from build123d import *

# Parameters (mm, degrees)
BOSS_EXTRUDE1_DEPTH      = 20
BOSS_EXTRUDE2_REACH      = 36.375
BOSS_EXTRUDE2_END_RADIUS = 102
BOSS_EXTRUDE2_START      = -9
SKETCH3_W                = 10
SKETCH3_H                = 2.5
SKETCH4_W                = 10
SKETCH4_H                = 2
BOSS_EXTRUDE3_DEPTH      = 10
CHAMFER2_SIZE            = 3
CHAMFER2_SIZE2           = 1.732050808
CHAMFER1_SIZE            = 4
CHAMFER1_SIZE2           = 2.309401077
SKETCH6_W                = 10
SKETCH6_H                = 1
BOSS_EXTRUDE4_DEPTH      = 0.2
CHAMFER3_SIZE            = 0.5


with BuildPart() as part:
    # Sketch2 → Boss-Extrude1 (new body)
    with BuildSketch(Plane(origin=(0, 0, 0), x_dir=(1, 0, 0), z_dir=(0, 1, 0))):
        with BuildLine():
            Line((-15.3, 1.977371993), (-15, 0))
            ThreePointArc((-15, 0), (0, 1.131400334), (15, 0))
            Line((15, 0), (15.3, 1.977371993))
            ThreePointArc((15.3, 1.977371993), (0, 3.131400334), (-15.3, 1.977371993))
        make_face()
    extrude(amount=BOSS_EXTRUDE1_DEPTH)

    # Boss-Extrude2: up to this cylinder (the profile starts outside it)
    boss_extrude2_end = Plane(origin=(0, 6.463137, 98.868599666), z_dir=(0, -1, 0)) * Cylinder(BOSS_EXTRUDE2_END_RADIUS, 277.75, mode=Mode.PRIVATE)
    # Sketch3 → Boss-Extrude2 (add, up to the surface)
    with BuildSketch(Plane.XY.offset(BOSS_EXTRUDE2_START), mode=Mode.PRIVATE) as boss_extrude2_sk1:
        with Locations((0, 6.463137396)):
            Rectangle(SKETCH3_W, SKETCH3_H)
    boss_extrude2_tool1 = extrude(boss_extrude2_sk1.sketch, amount=BOSS_EXTRUDE2_REACH, mode=Mode.PRIVATE) - boss_extrude2_end
    add(boss_extrude2_tool1.solids().sort_by_distance((0, 6.463137, -9))[0])

    # Sketch4 → Boss-Extrude3 (add)
    with BuildSketch(Plane(origin=(0, 7.713137396, 0), x_dir=(1, 0, 0), z_dir=(0, 1, 0))):
        with Locations((0, 8)):
            Rectangle(SKETCH4_W, SKETCH4_H)
    extrude(amount=BOSS_EXTRUDE3_DEPTH)

    # Chamfer2
    chamfer2_edges = [part.edges().sort_by_distance(p)[0] for p in [
        (0, 7.713137396, -7),
    ]]
    chamfer2_side = [part.faces().sort_by_distance(p)[0] for p in [
        (0, 12.713137396, -7),
    ]]
    chamfer(chamfer2_edges, length=CHAMFER2_SIZE, length2=CHAMFER2_SIZE2, reference=chamfer2_side[0])

    # Chamfer1
    chamfer1_edges = [part.edges().sort_by_distance(p)[0] for p in [
        (0, 5.213137396, -9),
    ]]
    chamfer1_side = [part.faces().sort_by_distance(p)[0] for p in [
        (0, 11.463137396, -9),
    ]]
    chamfer(chamfer1_edges, length=CHAMFER1_SIZE, length2=CHAMFER1_SIZE2, reference=chamfer1_side[0])

    # Sketch6 → Boss-Extrude4 (add)
    with BuildSketch(Plane.XY.offset(-7)):
        with Locations((0, 13.213137396)):
            Rectangle(SKETCH6_W, SKETCH6_H)
    extrude(amount=BOSS_EXTRUDE4_DEPTH)

    # Chamfer3
    # the kernel refuses this chamfer: 0.5 mm, written as the material it takes off along each edge
    with BuildSketch(Plane(origin=(-6.285841494, 13.713137396, -6.8), x_dir=(0, 0.027495876610585647, -0.9996219169112968), z_dir=(1, 0, 0))) as chamfer3_piece_1_section:
        Polygon((CHAMFER3_SIZE * 0.999621916911, -CHAMFER3_SIZE * 0.0274958766106), (-CHAMFER3_SIZE * 0.0274958766106, -CHAMFER3_SIZE * 0.999621916911), (0, 0), align=None)
    chamfer3_piece_1 = extrude(amount=12.571682988, mode=Mode.PRIVATE)
    chamfer3_piece_1 = split(chamfer3_piece_1, bisect_by=Plane(origin=(0, 13.506192151, -7), z_dir=(0, 0, 1)), keep=Keep.TOP, mode=Mode.PRIVATE)
    add(chamfer3_piece_1, mode=Mode.SUBTRACT)


solid = part.part
Source: CAD feature listing. Evaluate the final solid. Frame: model axes, mm. A direction names the side the tool comes from. Coordinates: 2 decimals unless noted, no trailing zeros. Order: outer loops, then holes, each group sorted by start corner. A loop starts at its lowest first (then second) coordinate and runs counter-clockwise, first axis right, second up.
Item 1: Cut plane A-A (y = 15). Return loops of the section in (x, z).
Output values:
outline: (-15.3, -1.98) arc R102 ccw to (15.3, -1.98) - (15, 0) arc R100 cw to (-15, 0) - close; (-5, -9) - (5, -9) - (5, -7) - (-5, -7) - close
Item 2: Material intervals for line 1 (Z direction, x = -1, y = 13.5); line 2 (Y direction, x = 1, z = -5.25); line 3 (X direction, y = 7.5, z = -4.75), sorted ascending.
Output values:
line 1: z = -9 to -7, -3.13 to -1.13
line 2: y = 5.21 to 7.71
line 3: x = -5 to 5
Item 3: Set-up query: faces 1 (the face through (-15.15, 9.86, -1)), 2 (the face through (5, 10, -7)), 3 (the face through (0, 17.713, -8)), 4 (the face through (0, 16, -7)). Return all of +Z, -Z, +X, -X, +Y, -Y with unobstructed straight access to the full face (end or side cutting, diameter ignored); none if empty.
Output values:
face 1: +Z, -X, +Y, -Y
face 2: -Z, +X, +Y, -Y
face 3: -Z, +X, -X, +Y
face 4: +X, -X, +Y
Item 4: Pull-direction query (Y, two-part tool) for faces 5 (the face through (0, 12, -7)), 6 (the face through (-5, 10, -7)), 7 (the face through (0, 20, -2)); classes: pulls with the +Y half, pulls with the -Y half, needs draft (parallel to the pull), parting line crosses it, or undercut.
Output values:
face 5: undercut
face 6: needs draft
face 7: pulls with the +Y half
Item 5: Cut plane D-D (y = 4). Return loops of the section in (x, z).
Output values:
outline: (-15.3, -1.98) arc R102 ccw to (15.3, -1.98) - (15, 0) arc R100 cw to (-15, 0) - close
Item 6: Cut plane B-B (z = -0.75). Return loops of the section in (x, y), plus the area to 3 significant figures.
Output values:
outline: (-15.11, 0) - (-8.73, 0) - (-8.73, 20) - (-15.11, 20) - close; (8.73, 0) - (15.11, 0) - (15.11, 20) - (8.73, 20) - close
area: 256 mm2
Item 7: Cut plane C-C (x = -3.5). Return loops of the section in (y, z), plus the area to 3 significant figures.
Output values:
outline: (0, -3.07) - (5.21, -3.07) - (5.21, -6.69) - (9.21, -9) - (17.71, -9) - (17.71, -7) - (13.41, -7) - (13.21, -6.8) - (12.71, -6.8) - (12.71, -7) - (10.71, -7) - (7.71, -5.27) - (7.71, -3.07) - (20, -3.07) - (20, -1.07) - (0, -1.07) - close
area: 72.9 mm2
Item 8: First-contact query: P1, Ø1, axis at x = -4, y = 15, coming from the +Z side; P2, Ø0.6, axis at x = 1.5, z = -8, coming from the +Y side; P3, Ø5, axis at y = 13, z = -7, coming from the -X side. Flat tips, straight axial feed; report the tip coordinate or a pass-through.
Output values:
P1: stops at z = -1.03
P2: stops at y = 17.71
P3: stops at x = -5
